The figure shows three views and two pictorial views of one solid part (mm, origin at its lowest corner). Answer the questions. Give positions to 0.01 mm unless a question says otherwise; leave off trailing zeros. Loops run counter-clockwise (first coordinate to the right, second up) from the corner with the lowest first, then second, coordinate; pieces in that order, holes last. Notation, with made-up numbers: M 2,88.25 L 24,88.25 A17 cw 24,117.25 Z; hole C 19,-30.75 d5. An arc over 180 degrees is marked long. Write item = value, one per line. Start each with the question number.
1. Consider L1, parallel to Z at x = 3.25, y = 270; L2, parallel to Y at x = 2.75, z = 10; L3, parallel to Y at x = 1.25, z = 12.5. Determine where each line is inside the solid, lowest interval first. Write a range as [from, to].
2. Section A-A on z = 10 is taken. Determine the outline of the cut face in (x, y).
3. Section B-B on y = 270 is taken. Determine the outline of the cut face in (x, z).
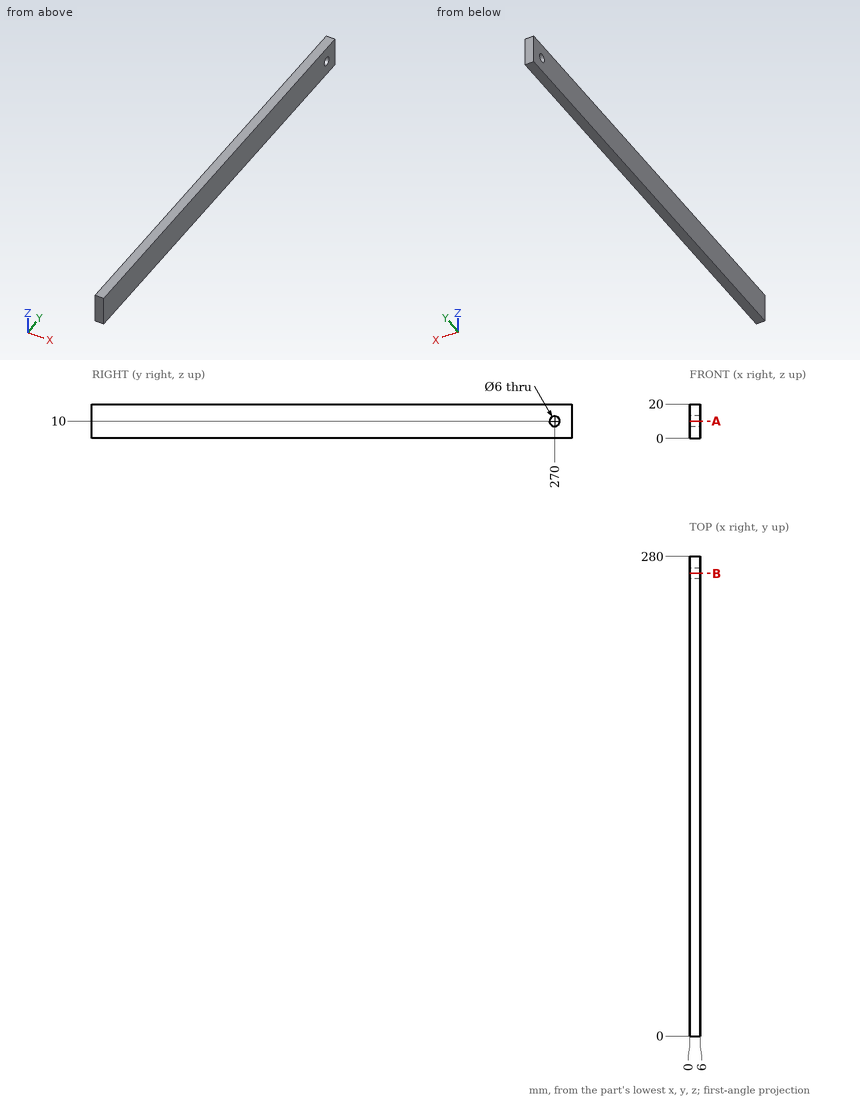
Verdict:
q1.L1 = [0, 7], [13, 20]
q1.L2 = [0, 267], [273, 280]
q1.L3 = [0, 268.34], [271.66, 280]
q2.outline = M 0,0 L 6,0 L 6,267 L 0,267 Z; M 0,273 L 6,273 L 6,280 L 0,280 Z
q3.outline = M 0,0 L 6,0 L 6,7 L 0,7 Z; M 0,13 L 6,13 L 6,20 L 0,20 Z
